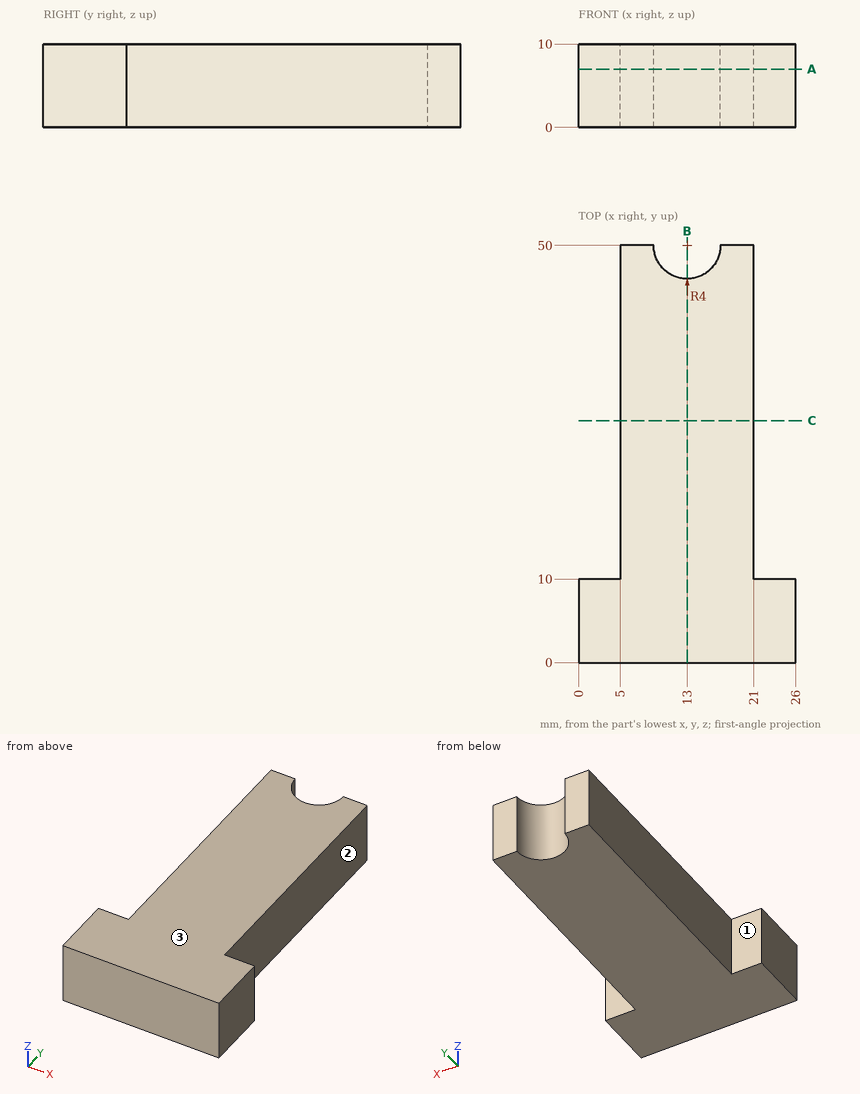
For this review, use the dimensioned drawing (mm, ordinates from the lowest corner) and the shaded views. A direction names the side the tool comes from. Round coordinates to 2 decimals unless told otherwise and drop trailing zeros. Write each loop counter-clockwise with the first axis right and the second up, starting at its lowest first coordinate (ties: lowest second). Pieces come first, ordered by that corner, then holes. Notation, with made-up numbers: (-34, 48.5) - (-2, 48.5) arc R29 ccw to (-2, 80.5) - close; hole circle Ø9 at (8, 33.5). An arc over 180 degrees is marked (long way). One line per item, written item: value. Start each with the question number.
1. Clearance check with flat-ended pins moving along their axes: P1, Ø5, axis at y = 36, z = 3, coming from the -X side; P2, Ø1, axis at y = 40, z = 6.5, coming from the +X side. State where each tip first meets the part, or that it passes through.
2. Machinability: for the marked faces 1, 2 and 3, which of the approach directions +Z, -Z, +X, -X, +Y, -Y give a long, thin tool a straight path to every point of the face, cutting with its end or side? Answer none if there is none.
3. To check wall thickness, follow L1, parallel to X at y = 12, z = 5.5; L2, parallel to X at y = 46.5, z = 6.25; L3, parallel to Y at x = 23.25, z = 1.75. State the ranges of each line that lie inside material, in increasing order. Write a range as from..to.
4. Consider section A-A on z = 7. Write out the cut boundary in (x, y), and give its area (3 significant figures).
5. Consider section C-C on y = 29. Write out the cut boundary in (x, z).
6. Consider section B-B on x = 13. Write out the cut boundary in (y, z).
Checks:
1. P1: stops at x = 5
1. P2: stops at x = 21
2. face 1: +Z, -Z, -X, +Y
2. face 2: +Z, -Z, +X, +Y
2. face 3: +Z, +X, -X, +Y, -Y
3. L1: x = 5..21
3. L2: x = 5..11.06, 14.94..21
3. L3: y = 0..10
4. outline: (0, 0) - (26, 0) - (26, 10) - (21, 10) - (21, 50) - (17, 50) arc R4 cw to (9, 50) - (5, 50) - (5, 10) - (0, 10) - close
4. area: 875 mm^2
5. outline: (5, 0) - (21, 0) - (21, 10) - (5, 10) - close
6. outline: (0, 0) - (46, 0) - (46, 10) - (0, 10) - close
